Here's how the part is built. I have some questions about the finished solid (model axes, mm). Face numbers are marked on the shaded views. Coordinates: 2 decimals unless noted, no trailing zeros. Write each loop counter-clockwise with the first axis right and the second up, starting at its lowest first coordinate (ties: lowest second). Pieces come first, ordered by that corner, then holes.
```python
from build123d import *

# Parameters (mm, degrees)
SKETCH_1_W           = 2
SKETCH_1_H           = 250
EXTRUDE_1_DEPTH      = 20
EXTRUDE_2_DEPTH      = 20
EXTRUDE_2_DEPTH_BACK = 40
SKETCH_2_W           = 20
SKETCH_2_H           = 2
SKETCH_3_R           = 1.51
CUT_EXTRUDE_1_DEPTH  = 254.818833029
FILLET_1_R           = 5
FILLET_2_RADIUS      = 10
FILLET_2_LENGTH      = 2
SKETCH_4_R           = 1.51
CUT_EXTRUDE_2_DEPTH  = 254.818833029


with BuildPart() as part:
    # 草图1 → 凸台-拉伸1 (new body)
    with BuildSketch(Plane.XY):
        with Locations((1, 125)):
            Rectangle(SKETCH_1_W, SKETCH_1_H)
    extrude(amount=EXTRUDE_1_DEPTH)

    # 草图2 → 凸台-拉伸2 (add, two sides: drawn at the far end of the back side and taken through both)
    with BuildSketch(Plane(origin=(0, 0, 0), x_dir=(-1, 0, 0), z_dir=(0, 0, -1)).offset(-EXTRUDE_2_DEPTH_BACK)):
        with Locations((8, -1)):
            Rectangle(SKETCH_2_W, SKETCH_2_H)
    extrude(amount=EXTRUDE_2_DEPTH + EXTRUDE_2_DEPTH_BACK)

    # 草图3 → 切除-拉伸1 (cut, through all)
    with BuildSketch(Plane(origin=(0, 0, 0), x_dir=(1, 0, 0), z_dir=(0, 1, 0))):
        with Locations(Location((-8, -25, 0), (0, 0, 270))):
            Circle(SKETCH_3_R)
        with Locations(Location((-8, -10, 0), (0, 0, 270))):
            Circle(SKETCH_3_R)
        with Locations(Location((-8, 5, 0), (0, 0, 90))):
            Circle(SKETCH_3_R)
    extrude(amount=-CUT_EXTRUDE_1_DEPTH, mode=Mode.SUBTRACT)

    # 圆角1
    fillet_1_edges = [part.edges().sort_by_distance(p)[0] for p in [
        (-18, -1, 40),
        (2, -1, 40),
        (2, -1, -20),
        (-18, -1, -20),
    ]]
    fillet(fillet_1_edges, radius=FILLET_1_R)

    # 圆角2: full round fillet: the end face becomes a half cylinder, R = half its width
    fillet_2_face = Plane((1, 250, 10), x_dir=(1, 0, 0), z_dir=(0, 1, 0))  # on the end face: x along it, z out of the body
    fillet_2_slab = fillet_2_face.offset(-FILLET_2_RADIUS / 2) * Box(FILLET_2_LENGTH, 2 * FILLET_2_RADIUS, FILLET_2_RADIUS, mode=Mode.PRIVATE)  # the body's end, R deep
    fillet_2_round = Plane((1, 240, 10), x_dir=(0, 1, 0), z_dir=(1, 0, 0)) * Cylinder(FILLET_2_RADIUS, FILLET_2_LENGTH, mode=Mode.PRIVATE)  # its axis R under the face
    add(fillet_2_slab - fillet_2_round, mode=Mode.SUBTRACT)

    # 草图4 → 切除-拉伸2 (cut, through all)
    with BuildSketch(Plane.ZY):
        with Locations((10, 240)):
            Circle(SKETCH_4_R)
        with Locations((10, 230)):
            Circle(SKETCH_4_R)
        with Locations((10, 220)):
            Circle(SKETCH_4_R)
        with Locations((10, 210)):
            Circle(SKETCH_4_R)
        with Locations((10, 200)):
            Circle(SKETCH_4_R)
        with Locations((10, 190)):
            Circle(SKETCH_4_R)
        with Locations((10, 180)):
            Circle(SKETCH_4_R)
        with Locations((10, 170)):
            Circle(SKETCH_4_R)
        with Locations((10, 160)):
            Circle(SKETCH_4_R)
        with Locations((10, 150)):
            Circle(SKETCH_4_R)
        with Locations((10, 140)):
            Circle(SKETCH_4_R)
    extrude(amount=-CUT_EXTRUDE_2_DEPTH, mode=Mode.SUBTRACT)


solid = part.part
```
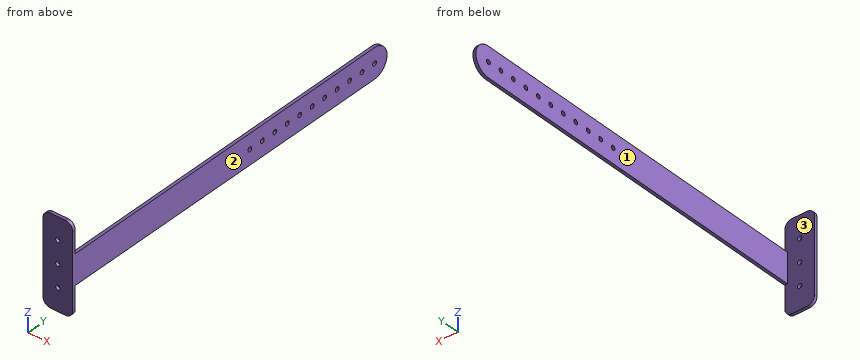
1) I need wall thicknesses on probe 1 along Z at (x, y) = (0.6, 230); probe 2 along X at (y, z) = (-1, 10); probe 3 along X at (y, z) = (125.5, 7). Which ranges of each line are inside material? Lowest first, please.
Values follow:
probe 1: z = 0 to 8.49, 11.51 to 20
probe 2: x = -18 to -9.51, -6.49 to 2
probe 3: x = 0 to 2
2) We'd pull the mould along X, two halves only. Please class the marked faces 1, 2 and 3: pulls with the +X half, pulls with the -X half, needs draft (parallel to the pull), parting line crosses it, or undercut.
Values follow:
face 1: pulls with the -X half
face 2: pulls with the +X half
face 3: needs draft
3) Will these pins go through, and if not, where does the flat tip stop? pin 1 (5 mm diameter, centred on y = 170, z = 10, fed in from -X); pin 2 (2.5 mm diameter, centred on y = 150, z = 10, fed in from -X); pin 3 (1 mm diameter, centred on x = -13, z = 4, fed in from +Y); pin 4 (1 mm diameter, centred on x = 1, y = 137.5, fed in from -Z).
Values follow:
pin 1: stops at x = 0
pin 2: passes through
pin 3: stops at y = 0
pin 4: stops at z = 0
4) Imagine slicing it at A-A on y = 76.5. Please give me the cut outline in (x, z), then the cut area to 3 significant figures.
Values follow:
outline: (0, 0) - (2, 0) - (2, 20) - (0, 20) - close
area: 40.0 mm2
